Print and shaded views of the part. All mm, measured from the part's lowest x, y and z. Coordinates: 2 decimals unless noted, no trailing zeros. Order: outer loops, then holes, each group sorted by start corner. A loop starts at its lowest first (then second) coordinate and runs counter-clockwise, first axis right, second up. Notation, with made-up numbers: (20, 28.25) - (50, 28.25) arc R29 ccw to (50, 61.25) - close; hole circle Ø2 at (51.5, -23). An arc over 180 degrees is marked (long way). Write each question's results on one line, items separated by ' | '.
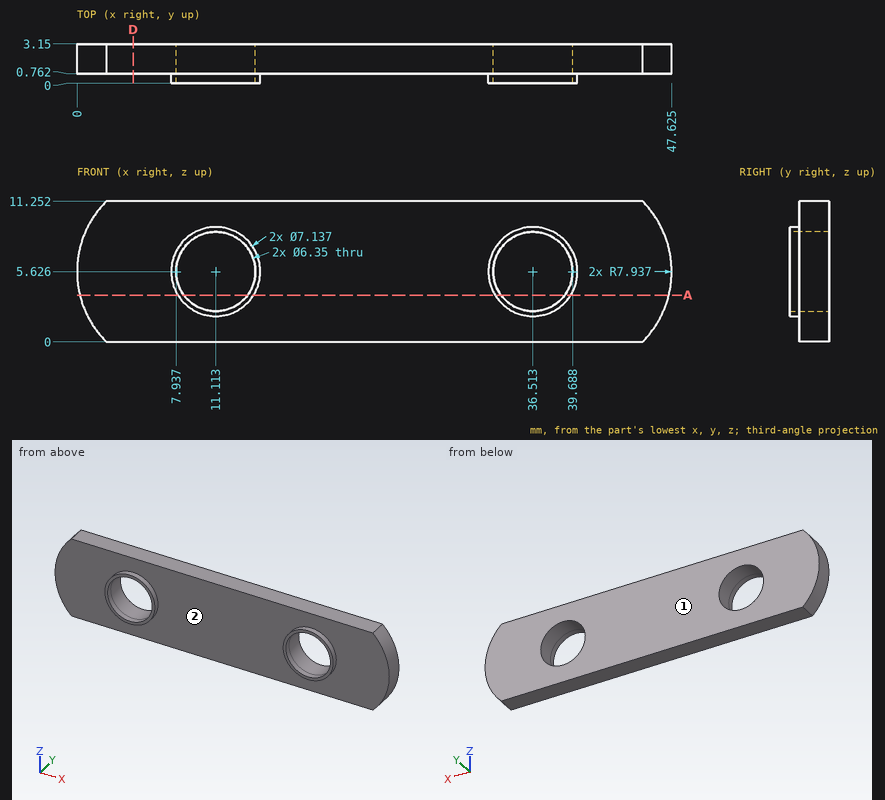
1. Two-plate mould, pull along X, no slides. Class the marked faces 1 and 2: +X half, -X half, draft (parallel to the pull), parting line (faces both ways), or undercut.
Solved:
face 1: draft | face 2: undercut
2. Band-saw the part on A-A on z = 3.75. Give the number of separate pieces and of enclosed holes in the cut face.
Solved:
separate pieces: 3 | enclosed holes: 0
3. Drop a flat-ended pin along its axis: pin 1 Ø5.5 at (x, z) = (36.51, 5.63) entering from +Y. Give the stop position or say it passes through.
Solved:
pin 1: passes through
4. Band-saw the part on D-D on x = 4.5. Give the cut face in (y, z).
Solved:
outline: (0.76, 0) - (3.15, 0) - (3.15, 11.25) - (0.76, 11.25) - close
5. Probe line 1 (X direction, y = 0.35, z = 5.75) (1 decimal); line 2 (X direction, y = 1.6, z = 5.75) (1 decimal); line 3 (X direction, y = 0.6, z = 6.25) (1 decimal). List the from-to ranges inside material, lowest first.
Solved:
line 1: x = 7.5 to 7.9, 14.3 to 14.7, 32.9 to 33.3, 39.7 to 40.1 | line 2: x = 0 to 7.9, 14.3 to 33.3, 39.7 to 47.6 | line 3: x = 7.6 to 8, 14.2 to 14.6, 33 to 33.4, 39.6 to 40
